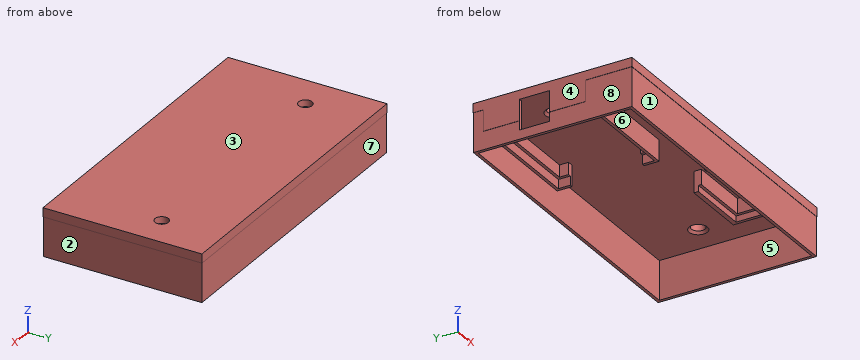
from build123d import *

# Parameters (mm, degrees)
SKETCH068_W         = 103
SKETCH068_H         = 53
PAD046_DEPTH        = 3
HOLE004_D           = 4.5
HOLE004_DEPTH       = 25
HOLE004_CSINK_D     = 6.1
HOLE004_CSINK_ANGLE = 90
PAD047_DEPTH        = 7
SKETCH071_W         = 102.8
SKETCH071_H         = 52.8
SKETCH071_W_2       = 100.8
SKETCH071_H_2       = 50.8
PAD048_DEPTH        = 13
PAD049_DEPTH        = 7
PAD050_DEPTH        = 5
PAD051_DEPTH        = 4
SKETCH076_W         = 10
SKETCH076_H         = 10
POCKET015_DEPTH     = 5


with BuildPart() as part:
    # Sketch068 → Pad046 (new body)
    with BuildSketch(Plane.XY):
        with Locations((51.5, 26.5)):
            Rectangle(SKETCH068_W, SKETCH068_H)
    extrude(amount=-PAD046_DEPTH)

    # Hole004
    with Locations(Plane(origin=(0, 0, -3), x_dir=(1, 0, 0), z_dir=(0, 0, -1))):
        with Locations((12, -33), (92, -33)):
            CounterSinkHole(HOLE004_D / 2, HOLE004_CSINK_D / 2, depth=HOLE004_DEPTH, counter_sink_angle=HOLE004_CSINK_ANGLE)

    # Sketch070 → Pad047 (join)
    with BuildSketch(Plane.XY.offset(-3)):
        Polygon((0, 49.5), (41, 49.5), (41, 44.5), (40, 44.5), (40, 48.5), (1, 48.5), (1, 16.5), (40, 16.5), (40, 20.5), (41, 20.5), (41, 15.5), (0, 15.5), align=None)
    extrude(amount=-PAD047_DEPTH)

    # Sketch071 → Pad048 (join)
    with BuildSketch(Plane.XY.offset(-3)):
        with Locations((51.5, 26.5)):
            Rectangle(SKETCH071_W, SKETCH071_H)
        with Locations((51.5, 26.5)):
            Rectangle(SKETCH071_W_2, SKETCH071_H_2, mode=Mode.SUBTRACT)
    extrude(amount=-PAD048_DEPTH)

    # Sketch073 → Pad049 (join)
    with BuildSketch(Plane.XY.offset(-3)):
        Polygon((52, 1), (84, 1), (84, 16.5), (62, 16.5), (62, 15), (83, 15), (83, 2), (53, 2), (53, 7), (52, 7), align=None)
    extrude(amount=-PAD049_DEPTH)

    # Sketch074 → Pad050 (join)
    with BuildSketch(Plane.XY.offset(-3)):
        Polygon((53, 7), (53, 2), (83, 2), (83, 15), (62, 15), (62, 14), (82, 14), (82, 3), (54, 3), (54, 7), align=None)
    extrude(amount=-PAD050_DEPTH)

    # Sketch075 → Pad051 (join)
    with BuildSketch(Plane.XY.offset(-3)):
        Polygon((40, 20.5), (39, 20.5), (39, 17.5), (1.1, 17.5), (1.1, 16.5), (40, 16.5), align=None)
        Polygon((40, 44.5), (40, 48.5), (1.1, 48.5), (1.1, 47.5), (39, 47.5), (39, 44.5), align=None)
    extrude(amount=-PAD051_DEPTH)

    # Sketch076 → Pocket015 (cut)
    with BuildSketch(Plane.YZ):
        with Locations((32.5, -8)):
            Rectangle(SKETCH076_W, SKETCH076_H)
    extrude(amount=POCKET015_DEPTH, mode=Mode.SUBTRACT)


with BuildPart() as part_1:
    # Body020 placement: moved
    add(part.part.moved(Location((3, 3, 17))))


solid = part_1.part
Work out the finished part from the listing and answer in its coordinate system (mm). Face numbers are marked on the shaded views. A direction names the side the tool comes from. Give positions to 0.01 mm unless a question says otherwise; leave off trailing zeros. Write each loop counter-clockwise with the first axis right and the second up, starting at its lowest first coordinate (ties: lowest second). Pieces come first, ordered by that corner, then holes. Notation, with made-up numbers: M 3,3.25 L 24,3.25 A17 ccw 24,14.25 Z; hole C 83,29.25 d8. An arc over 180 degrees is marked long. Answer as CSV lines item,"result".
Q1. The mould has two halves that part along X. Classify the marked faces 6, 7 and 8: +X half, -X half, draft (parallel to the pull), parting line (faces both ways), or undercut.
A:
face 6,"undercut"
face 7,"draft"
face 8,"-X half"
Q2. A cutting plane is placed at D-D on y = 11. Write down the section's boundary in (x, z).
A:
outline,"M 3,14 L 3.1,14 L 3.1,1 L 4.1,1 L 4.1,14 L 85,14 L 85,9 L 86,9 L 86,7 L 87,7 L 87,14 L 104.9,14 L 104.9,1 L 105.9,1 L 105.9,14 L 106,14 L 106,17 L 3,17 Z"
Q3. A cutting plane is placed at B-B on x = 95. Write down the section's boundary in (y, z), plus the area to 3 significant figures.
A:
outline,"M 3,14 L 3.1,14 L 3.1,1 L 4.1,1 L 4.1,14 L 32.95,14 L 33.75,14.8 L 33.75,17 L 3,17 Z; M 38.25,14.8 L 39.05,14 L 54.9,14 L 54.9,1 L 55.9,1 L 55.9,14 L 56,14 L 56,17 L 38.25,17 Z"
area,"171 mm²"
Q4. Given P1, Ø6, axis at x = 42, z = 9, coming from the -Y side; P2, Ø2, axis at y = 7.5, z = 7.5, coming from the +X side; P3, Ø2, axis at x = 42, z = 4, coming from the +Y side, each flat-ended and moving along its own axis, determine where each tip first touches the part or whether it passes through.
A:
P1,"stops at y = 3.1"
P2,"stops at x = 105.9"
P3,"stops at y = 55.9"
Q5. Find the intervals of material crossed by probe 1 along Y at (x, z) = (71, 10.5); probe 2 along X at (y, z) = (36, 15.35); probe 3 along Y at (x, z) = (19, 7.5), in increasing order. Write a range as [from, to].
A:
probe 1,"y = [3.1, 6], [17, 19.5], [54.9, 55.9]"
probe 2,"x = [3, 12.75], [17.25, 92.75], [97.25, 106]"
probe 3,"y = [3.1, 4.1], [18.5, 19.5], [51.5, 52.5], [54.9, 55.9]"
Q6. A tool of negligible diameter and unlimited length cuts with its end or side. For the marked faces 1, 2, 3, 4 and 5, from which of +Z, -Z, +X, -X, +Y, -Y can it reach the whole face along a straight path? Write none if from no direction.
A:
face 1,"-Z, +X, -X, -Y"
face 2,"-Z, +X, +Y, -Y"
face 3,"+Z, +X, -X, +Y, -Y"
face 4,"+Z, -Z, -X, +Y, -Y"
face 5,"-Z"
Q7. A cutting plane is placed at C-C on z = 2.75. Write down the section's boundary in (x, y), plus the area to 3 significant figures.
A:
outline,"M 3.1,3.1 L 105.9,3.1 L 105.9,55.9 L 3.1,55.9 Z; hole M 4.1,4.1 L 104.9,4.1 L 104.9,54.9 L 4.1,54.9 Z"
area,"307 mm²"
Q8. A cutting plane is placed at A-A on y = 36. Write down the section's boundary in (x, z), plus the area to 3 significant figures.
A:
outline,"M 3,14 L 11.95,14 L 12.75,14.8 L 12.75,17 L 3,17 Z; M 3.1,1 L 4.1,1 L 4.1,4 L 3.1,4 Z; M 17.25,14.8 L 18.05,14 L 91.95,14 L 92.75,14.8 L 92.75,17 L 17.25,17 Z; M 97.25,14.8 L 98.05,14 L 104.9,14 L 104.9,1 L 105.9,1 L 105.9,14 L 106,14 L 106,17 L 97.25,17 Z"
area,"297 mm²"
